For this review, take the finished solid that the model builds, in its own axes (mm). Round coordinates to 2 decimals unless told otherwise and drop trailing zeros. Order: outer loops, then holes, each group sorted by start corner. A loop starts at its lowest first (then second) coordinate and runs counter-clockwise, first axis right, second up. Notation, with made-up numbers: (-36, 71) -> (5, 71) arc R16 cw to (5, 91) -> close; hole circle Ø11 at (24, 11). An arc over 180 degrees is marked (long way). Answer in a Markdown table with one row per item.
```python
from build123d import *

# Parameters (mm, degrees)
BOSS_EXTRUDE1_DEPTH             = 3.175
F_5_32_0_15625_DIAMETER_HOLE1_D = 3.96875
FILLET1_R                       = 12.7


with BuildPart() as part:
    # Sketch1 → Boss-Extrude1 (new body)
    with BuildSketch(Plane(origin=(0, 0, 0), x_dir=(1, 0, 0), z_dir=(0, 1, 0))):
        with BuildLine():
            Line((-58.261140344, 73.958269638), (-59.57789635, 162.152192036))
            Line((-59.57789635, 162.152192036), (-46.350471986, 198.78134649))
            ThreePointArc((-46.350471986, 198.78134649), (0, 209.411849995), (46.350471986, 198.78134649))
            Line((46.350471986, 198.78134649), (59.57789635, 162.152192036))
            Line((59.57789635, 162.152192036), (58.261140344, 73.958269638))
            Line((58.261140344, 73.958269638), (43.887596105, 48.613026492))
            Line((43.887596105, 48.613026492), (27.448255842, 1.5875))
            Line((27.448255842, 1.5875), (-27.448255842, 1.5875))
            Line((-27.448255842, 1.5875), (-43.887596105, 48.613026492))
            Line((-43.887596105, 48.613026492), (-58.261140344, 73.958269638))
        make_face()
    extrude(amount=BOSS_EXTRUDE1_DEPTH)

    # 5/32 (0.15625) Diameter Hole1 (through all)
    with Locations(Plane(origin=(0, 3.175, 0), x_dir=(1, 0, 0), z_dir=(0, 1, 0))):
        with Locations((0, 6.48335), (-35.45205, 194.449583064), (35.45205, 194.449583064)):
            Hole(F_5_32_0_15625_DIAMETER_HOLE1_D / 2)

    # Fillet1
    fillet1_edges = [part.edges().sort_by_distance(p)[0] for p in [
        (-59.57789635, 1.5875, -162.152192036),
        (-58.261140344, 1.5875, -73.958269638),
        (-43.887596105, 1.5875, -48.613026492),
        (-27.448255842, 1.5875, -1.5875),
        (27.448255842, 1.5875, -1.5875),
        (43.887596105, 1.5875, -48.613026492),
        (58.261140344, 1.5875, -73.958269638),
        (59.57789635, 1.5875, -162.152192036),
        (46.350471986, 1.5875, -198.78134649),
        (-46.350471986, 1.5875, -198.78134649),
    ]]
    fillet(fillet1_edges, radius=FILLET1_R)


solid = part.part
```
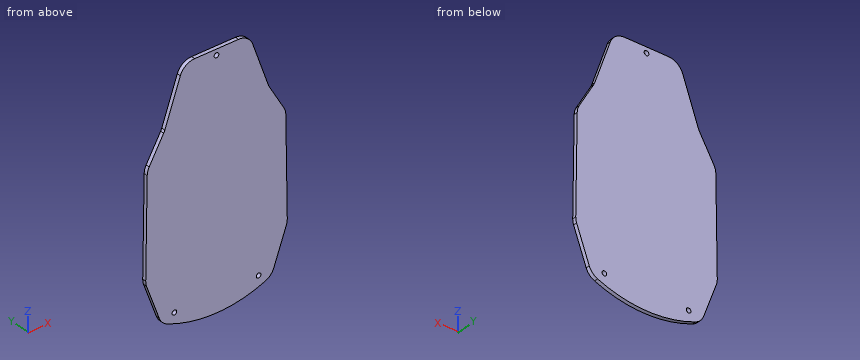
Q1. Clearance check with flat-ended pins moving along their axes: pin 1 Ø1.5 at (y, z) = (0.5, -155.5) entering from +X; pin 2 Ø1.5 at (y, z) = (1.5, -101.5) entering from +X; pin 3 Ø3 at (x, z) = (-35.45, -194.45) entering from -Y. State where each tip first meets the part, or that it passes through.
Answer key:
| item | result |
|---|---|
| pin 1 | stops at x = 59.49 |
| pin 2 | stops at x = 58.68 |
| pin 3 | passes through |
Q2. Take a section at D-D, the plane z = -67.5. Write out the cut boundary in (x, y) (3 decimals).
Answer key:
| item | result |
|---|---|
| outline | (-54.599, 0) -> (54.599, 0) -> (54.599, 3.175) -> (-54.599, 3.175) -> close |
Q3. Take a section at B-B, the plane y = 2.6. Write out the cut boundary in (x, z) (1 decimal).
Answer key:
| item | result |
|---|---|
| outline | (-59.5, -159.8) arc R12.7 ccw to (-58.8, -164.3) -> (-48.2, -193.7) arc R12.7 ccw to (-41.1, -201.1) arc R106.4 ccw to (41.1, -201.1) arc R12.7 ccw to (48.2, -193.7) -> (58.8, -164.3) arc R12.7 ccw to (59.5, -159.8) -> (58.3, -77.2) arc R12.7 ccw to (56.7, -71.1) -> (44.5, -49.6) arc R12.7 cw to (43.5, -47.5) -> (30.4, -10.1) arc R12.7 ccw to (18.4, -1.6) -> (-18.4, -1.6) arc R12.7 ccw to (-30.4, -10.1) -> (-43.5, -47.5) arc R12.7 cw to (-44.5, -49.6) -> (-56.7, -71.1) arc R12.7 ccw to (-58.3, -77.2) -> close; hole circle Ø4 at (-35.5, -194.4); hole circle Ø4 at (0, -6.5); hole circle Ø4 at (35.5, -194.4) |
Q4. Take a section at C-C, the plane z = -95.5. Write out the cut boundary in (x, y) (3 decimals), then the cut area to 3 significant figures.
Answer key:
| item | result |
|---|---|
| outline | (-58.583, 0) -> (58.583, 0) -> (58.583, 3.175) -> (-58.583, 3.175) -> close |
| area | 372 mm^2 |
Q5. Take a section at A-A, the plane x = 0. Write out the cut boundary in (y, z) (1 decimal).
Answer key:
| item | result |
|---|---|
| outline | (0, -209.4) -> (3.2, -209.4) -> (3.2, -8.5) -> (0, -8.5) -> close; (0, -4.5) -> (3.2, -4.5) -> (3.2, -1.6) -> (0, -1.6) -> close |
Q6. To check wall thickness, follow probe 1 along Z at (x, y) = (-2.5, 0.45); probe 2 along X at (y, z) = (0.35, -120); probe 3 along X at (y, z) = (0.9, -200). State the ranges of each line that lie inside material, in increasing order.
Answer key:
| item | result |
|---|---|
| probe 1 | z = -209.38 to -1.59 |
| probe 2 | x = -58.95 to 58.95 |
| probe 3 | x = -43.26 to 43.26 |
